The listing builds one solid part. Answer for the finished solid, in the listing's coordinates (mm). Face numbers are marked on the shaded views. A direction names the side the tool comes from. Give positions to 0.01 mm unless a question says otherwise; leave off trailing zeros. Write each loop counter-clockwise with the first axis right and the second up, starting at its lowest first coordinate (ties: lowest second). Pieces come first, ordered by that corner, then holes. Notation, with made-up numbers: (41, 72) -> (47, 72) arc R21 ccw to (47, 96) -> close; hole circle Ø1 at (17.25, 3). An arc over 180 degrees is marked (long way). Put each result on its own line as item: value. Start each with the question number.
1) For a pull along X with two mould halves and no side action, classify the marked faces 3, 4, 5 and 6 as released by +X, released by -X, zero draft, split by the parting line, or undercut.
2) A cutting plane is placed at C-C (z = -1.25). Write down the section's boundary in (x, y), then the cut area to 3 significant figures.
3) A cutting plane is placed at A-A (x = 1.5). Write down the section's boundary in (y, z).
4) A cutting plane is placed at B-B (z = 3). Write down the section's boundary in (x, y), then the cut area to 3 significant figures.
5) Flat-ended cylindrical pins translate along their axes: pin 1 Ø1.5 at (y, z) = (2, 3.5) entering from +X; pin 2 Ø7 at (x, y) = (-3, -3) entering from +Z; pin 3 Ø0.9 at (x, z) = (-2.5, 3.5) entering from -Y. Find the tip coordinate at first contact, or state that the pin passes through.
6) A cutting plane is placed at D-D (y = -3). Write down the section's boundary in (x, z), then the cut area to 3 significant figures.
7) For the marked faces 1 and 2, determine the directions among +Z, -Z, +X, -X, +Y, -Y from which every point of the face is accessible in a straight line to the end or side of a thin tool.
8) Find the intervals of material crossed by line 1 along X through (y, z) = (1, 2.75); line 2 along Y through (x, z) = (6, 3.5); line 3 along X through (y, z) = (-2.5, 4.25), in increasing order. Write a range as from..to.
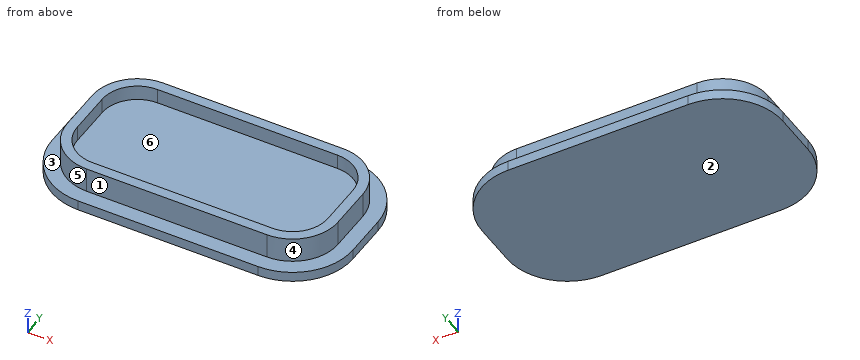
from build123d import *

# Parameters (mm, degrees)
F0_W     = 53.8
F0_H     = 26.7
F1_DEPTH = 5
F2_R     = 9
F3_T     = -2
F5_DEPTH = 2


with BuildPart() as f1:
    # F0 (on Top) → F1 (new body)
    with BuildSketch(Plane.XY):
        with Locations((-9.468303, 2.791487)):
            Rectangle(F0_W, F0_H)
    extrude(amount=F1_DEPTH)

    # F2
    f2_edges = [f1.edges().sort_by_distance(p)[0] for p in [
        (-36.368303, 16.141487, 2.5),
        (17.431697, 16.141487, 2.5),
        (17.431697, -10.558513, 2.5),
        (-36.368303, -10.558513, 2.5),
    ]]
    fillet(f2_edges, radius=F2_R)

    # F3
    f3_openings = [f1.faces().sort_by_distance(p)[0] for p in [
        (-9.468303, 2.791487, 5),
    ]]
    offset(amount=F3_T, openings=f3_openings)

    # F4 (on face) → F5 (join)
    with BuildSketch(Plane(origin=(0, 0, 0), x_dir=(1, 0, 0), z_dir=(0, 0, -1))):
        with BuildLine():
            Line((20.431697, -7.141487), (20.431697, 1.558513))
            ThreePointArc((20.431697, 1.558513), (16.916978, 10.043794), (8.431697, 13.558513))
            Line((8.431697, 13.558513), (-27.368303, 13.558513))
            ThreePointArc((-27.368303, 13.558513), (-35.853585, 10.043794), (-39.368303, 1.558513))
            Line((-39.368303, 1.558513), (-39.368303, -7.141487))
            ThreePointArc((-39.368303, -7.141487), (-35.853585, -15.626768), (-27.368303, -19.141487))
            Line((-27.368303, -19.141487), (8.431697, -19.141487))
            ThreePointArc((8.431697, -19.141487), (16.916978, -15.626768), (20.431697, -7.141487))
        make_face()
        with BuildLine():
            Line((17.431697, 1.558513), (17.431697, -7.141487))
            ThreePointArc((17.431697, -7.141487), (14.795658, -13.505448), (8.431697, -16.141487))
            Line((8.431697, -16.141487), (-27.368303, -16.141487))
            ThreePointArc((-27.368303, -16.141487), (-33.732264, -13.505448), (-36.368303, -7.141487))
            Line((-36.368303, -7.141487), (-36.368303, 1.558513))
            ThreePointArc((-36.368303, 1.558513), (-33.732264, 7.922474), (-27.368303, 10.558513))
            Line((-27.368303, 10.558513), (8.431697, 10.558513))
            ThreePointArc((8.431697, 10.558513), (14.795658, 7.922474), (17.431697, 1.558513))
        make_face(mode=Mode.SUBTRACT)
        with BuildLine():
            ThreePointArc((8.431697, -16.141487), (14.795658, -13.505448), (17.431697, -7.141487))
            Line((17.431697, -7.141487), (17.431697, 1.558513))
            ThreePointArc((17.431697, 1.558513), (14.795658, 7.922474), (8.431697, 10.558513))
            Line((8.431697, 10.558513), (-27.368303, 10.558513))
            ThreePointArc((-27.368303, 10.558513), (-33.732264, 7.922474), (-36.368303, 1.558513))
            Line((-36.368303, 1.558513), (-36.368303, -7.141487))
            ThreePointArc((-36.368303, -7.141487), (-33.732264, -13.505448), (-27.368303, -16.141487))
            Line((-27.368303, -16.141487), (8.431697, -16.141487))
        make_face()
    extrude(amount=F5_DEPTH)


solid = f1.part
Reply:
1. face 3: zero draft
1. face 4: released by +X
1. face 5: released by -X
1. face 6: undercut
2. outline: (-39.37, -1.56) arc R12 ccw to (-27.37, -13.56) -> (8.43, -13.56) arc R12 ccw to (20.43, -1.56) -> (20.43, 7.14) arc R12 ccw to (8.43, 19.14) -> (-27.37, 19.14) arc R12 ccw to (-39.37, 7.14) -> close
2. area: 1,830 mm2
3. outline: (-13.56, -2) -> (19.14, -2) -> (19.14, 0) -> (16.14, 0) -> (16.14, 5) -> (14.14, 5) -> (14.14, 2) -> (-8.56, 2) -> (-8.56, 5) -> (-10.56, 5) -> (-10.56, 0) -> (-13.56, 0) -> close
4. outline: (-36.37, -1.56) arc R9 ccw to (-27.37, -10.56) -> (8.43, -10.56) arc R9 ccw to (17.43, -1.56) -> (17.43, 7.14) arc R9 ccw to (8.43, 16.14) -> (-27.37, 16.14) arc R9 ccw to (-36.37, 7.14) -> close; hole (-34.37, -1.56) arc R7 ccw to (-27.37, -8.56) -> (8.43, -8.56) arc R7 ccw to (15.43, -1.56) -> (15.43, 7.14) arc R7 ccw to (8.43, 14.14) -> (-27.37, 14.14) arc R7 ccw to (-34.37, 7.14) -> close
4. area: 279 mm2
5. pin 1: stops at x = 17.43
5. pin 2: stops at z = 2
5. pin 3: stops at y = -10.56
6. outline: (-39.28, -2) -> (20.34, -2) -> (20.34, 0) -> (17.32, 0) -> (17.32, 5) -> (15.28, 5) -> (15.28, 2) -> (-34.22, 2) -> (-34.22, 5) -> (-36.25, 5) -> (-36.25, 0) -> (-39.28, 0) -> close
6. area: 239 mm2
7. face 1: +Z, +X, -X, -Y
7. face 2: -Z, +X, -X, +Y, -Y
8. line 1: x = -36.37..-34.37, 15.43..17.43
8. line 2: y = -10.56..-8.56, 14.14..16.14
8. line 3: x = -36.32..-34.3, 15.37..17.38
